Verification items for the finished model (mm, model axes). Face numbers are marked on the shaded views. A direction names the side the tool comes from. Coordinates: 2 decimals unless noted, no trailing zeros. Order: outer loops, then holes, each group sorted by start corner. A loop starts at its lowest first (then second) coordinate and runs counter-clockwise, first axis right, second up. Notation, with made-up numbers: (27.5, -30) -> (64.5, -30) arc R17 cw to (64.5, -2) -> close; hole circle Ø9 at (-12, 26). An arc over 180 degrees is marked (long way). Write item = value, one per line. Start each with the question number.
1. Go/stop test with flat-tipped pins: P1, Ø2, axis at x = 26.5, z = -5, coming from the -Y side; P2, Ø2, axis at x = 8.5, z = 4, coming from the +Y side; P3, Ø1.3, axis at y = -8.5, z = -2, coming from the +X side. Record where each tip stops, or that it passes through.
2. Thickness scan on line 1 along X through (y, z) = (6.75, 5); line 2 along Z through (x, y) = (20, -7); line 3 along Y through (x, z) = (28, 5.25). Record the ranges inside material, lowest first. Write a range as from..to.
3. Set-up check for the marked faces 4, 5 and 6: record each of +Z, -Z, +X, -X, +Y, -Y from which the full face is reachable in a straight line by a thin tool's end or side.
4. Cross-section at A-A on x = 22. Record the cut outline in (y, z).
5. Cross-section at B-B on x = 13.5. Record the cut outline in (y, z).
6. Release check for a two-part mould opening along X. For the marked faces 1, 2 and 3 record: +X half, -X half, draft (parallel to the pull), parting line (faces both ways), or undercut.
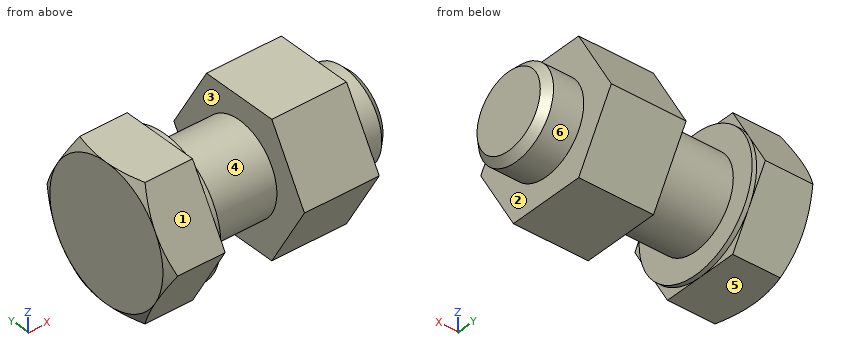
from build123d import *

# Parameters (mm, degrees)
BASEHEAD_DEPTH      = 7.76
SKETCH4_W           = 0.6
SKETCH4_H           = 11.392304845
BOSS_EXTRUDE1_DEPTH = 10


# Read off the part's stored shape, not the designer's step: HeadChamfer
with BuildPart() as part:
    # Sketch1 → BaseHead (new body)
    with BuildSketch(Plane(origin=(0, 0, 0), x_dir=(0, 0, -1), z_dir=(1, 0, 0))):
        Polygon((9, 5.196152423), (9, -5.196152423), (0, -10.392304845), (-9, -5.196152423), (-9, 5.196152423), (0, 10.392304845), align=None)
    extrude(amount=BASEHEAD_DEPTH)

    # HeadChamfer outline → HeadChamfer (revolve, cut)
    with BuildSketch(Plane.YX):
        Polygon((10.392304847, 0.803847578), (9, 0), (10.392304847, 0), align=None)
    revolve(axis=Axis((0, 0, 0), (1, 0, 0)), mode=Mode.SUBTRACT)

    # HeadChamfer 2 outline → HeadChamfer 2 (revolve)
    with BuildSketch(Plane.YX):
        Polygon((6, 7.76), (6, 31.796), (5.036, 32.76), (0, 32.76), (0, 7.76), align=None)
    revolve(axis=Axis((0, 0, 0), (1, 0, 0)))

    # Sketch4 → BearingFace (revolve, cut)
    with BuildSketch(Plane.XY, mode=Mode.PRIVATE) as bearingface_sk:
        with Locations((7.46, 14.696152423)):
            Rectangle(SKETCH4_W, SKETCH4_H)
    revolve(bearingface_sk.sketch.rotate(Axis((0, 0, 0), (1, 0, 0)), 90), axis=Axis((0, 0, 0), (1, 0, 0)), mode=Mode.SUBTRACT)

    # Sketch5 → Boss-Extrude1 (add)
    with BuildSketch(Plane(origin=(27.76, 0, 0), x_dir=(0, 0, -1), z_dir=(1, 0, 0))):
        Polygon((0, 10.392304845), (-9, 5.196152423), (-9, -5.196152423), (0, -10.392304845), (9, -5.196152423), (9, 5.196152423), align=None)
    extrude(amount=-BOSS_EXTRUDE1_DEPTH)


solid = part.part
Worked out:
q1.P1 = -8.08
q1.P2 = 8.36
q1.P3 = 27.76
q2.line_1 = 0..7.76, 17.76..27.76
q2.line_2 = -5.88..5.88
q2.line_3 = -2.9..2.9
q3.face_4 = none
q3.face_5 = -Z, +X, -X, +Y, -Y
q3.face_6 = +X
q4.outline = (-10.39, 0) -> (-5.2, -9) -> (5.2, -9) -> (10.39, 0) -> (5.2, 9) -> (-5.2, 9) -> close
q5.outline = circle Ø12 at (0, 0)
q6.face_1 = draft
q6.face_2 = +X half
q6.face_3 = undercut
